```python
from build123d import *

# Parameters (mm, degrees)
F3_R = 7.62
F4_R = 0.889


# Not quite as in the source:
# - a fillet or chamfer that OpenCascade refuses, or shapes differently, is made with other operations: its cross-section is extruded or revolved along the edge and cut away or added


with BuildPart() as f1:
    # F0 (on Front) → F1 (revolve)
    with BuildSketch(Plane.XZ):
        Polygon((-25.146, 6.35), (-25.146, 0), (-19.304, 0), (-19.304, 11.43), (-31.496, 9.525), (-31.496, 6.35), align=None)
    revolve(axis=Axis((0, 0, 48.3202852037), (0, 0, 1)))

    # F2: chamfer of 3.175 on 1 edges, made by hand

    # F2_s1 → F2_t2 (revolve, cut)
    with BuildSketch(Plane.XZ):
        Polygon((-28.3590617928, 10.0151465949), (-31.496, 6.35), (-31.496, 9.525), align=None)
    revolve(axis=Axis((0, 0, 9.525), (0, 0, 1)), mode=Mode.SUBTRACT)

    # F3
    f3_edges = [f1.edges().sort_by_distance(p)[0] for p in [
        (28.359062, 0, 10.015147),
    ]]
    fillet(f3_edges, radius=F3_R)

    # F4
    f4_edges = [f1.edges().sort_by_distance(p)[0] for p in [
        (19.304, 0, 11.43),
        (19.304, 0, 0),
        (25.146, 0, 0),
    ]]
    fillet(f4_edges, radius=F4_R)


solid = f1.part
```
Read the model definition and answer for the solid it produces. Units are mm, in the model's axes. Give positions to 0.01 mm unless a question says otherwise; leave off trailing zeros. Write each loop counter-clockwise with the first axis right and the second up, starting at its lowest first coordinate (ties: lowest second). Pieces come first, ordered by that corner, then holes. Notation, with made-up numbers: (20.25, 24.5) -> (59.25, 24.5) arc R11 cw to (59.25, 28.5) -> close; hole circle Ø9 at (69, 85). An arc over 180 degrees is marked (long way). Answer in a Markdown table with one row per item.
1) Straight lines are drawn through the part: line 1 (X direction, y = 0, z = 5); line 2 (X direction, y = 15, z = 9). For each, find the intervals that lie inside material, in ascending order. Write a range as [from, to].
Results list:
| item | result |
|---|---|
| line 1 | [-25.15, -19.3], [19.3, 25.15] |
| line 2 | [-24.81, -12.15], [12.15, 24.81] |
2) Each of these flat-tipped pins is pushed along its axis until it touches: pin 1 Ø4 at (x, y) = (-12, -22.5) entering from +Z; pin 2 Ø1.5 at (x, z) = (-19.5, 6.5) entering from -Y; pin 3 Ø1 at (x, z) = (-14, 6.5) entering from -Y. Where does it stop, or does it pass through?
Results list:
| item | result |
|---|---|
| pin 1 | z = 10.77 |
| pin 2 | y = -25.3 |
| pin 3 | y = -28.45 |
3) Section A-A on z = 1.75 is taken. Give the vertices of the cut face in (x, y).
Results list:
| item | result |
|---|---|
| outline | circle Ø50.29 at (0, 0); hole circle Ø38.61 at (0, 0) |
4) Determine the mould class of faces 1 (the conical face through (-19.08, 7.91, 11.22)), 2 (the cylindrical face through (-17.832, 7.394, 5.707)), 3 (the flat face through (6, -20, 0)) for opening direction X: released by +X, released by -X, zero draft, split by the parting line, or undercut.
Results list:
| item | result |
|---|---|
| face 1 | split by the parting line |
| face 2 | undercut |
| face 3 | zero draft |
